Geometry check sheet. Reference: the model listing, model coordinates, mm. A direction names the side the tool comes from. Give positions to 0.01 mm unless a question says otherwise; leave off trailing zeros. Order: outer loops, then holes, each group sorted by start corner. A loop starts at its lowest first (then second) coordinate and runs counter-clockwise, first axis right, second up. Notation, with made-up numbers: M 54,33 L 84,33 A5 ccw 84,38 Z; hole C 19.5,1.25 d1. An arc over 180 degrees is marked long. Put each result on its own line as item: value. Start each with the question number.
Q1. Section check C-C on z = 10. State how many separate pieces and enclosed holes the cut face has, then the cut area to 3 significant figures.
Q2. Go/stop test with flat-tipped pins: pin 1 (10 mm diameter, centred on y = 134.5, z = 5, fed in from -X); pin 2 (8.5 mm diameter, centred on x = 9.5, y = 96, fed in from -Z). Record where each tip stops, or that it passes through.
Q3. Access from +Z, -Z, +X, -X, +Y, -Y to the whole of each face (thin tool, end or side, straight path). Record for faces 1 (the flat face through (89, 63, 10)), 2 (the flat face through (49, 0, 10)), 3 (the flat face through (49, 197.5, 9)).
Q4. Material ranges on L1, parallel to Y at x = 42.5, z = 14.5; L2, parallel to X at y = 33, z = 9.25; L3, parallel to X at y = 104.5, z = 6.5, recorded low to high.
Q5. Section check B-B on x = 72. Record the cut outline in (y, z).
Q6. Section check A-A on y = 178. Record the cut outline in (x, z), then the cut area to 3 significant figures.
Q7. Mould release check, pull along Z, two halves, no side actions. Record for faces 4 (the cylindrical face through (2.535, 37.754, 10.165)), 5 (the flat face through (16, 124, 20)), 6 (the flat face through (11, 63, 10)): +Z half, -Z half, draft (parallel to the pull), parting line (faces both ways), or undercut.
```python
from build123d import *

# Parameters (mm, degrees)
F0_W        = 100
F0_H        = 200
F0_W_2      = 12
F0_H_2      = 43
F0_W_3      = 56
F0_H_3      = 180
F1_DEPTH    = 20
F2_R        = 3.75
F3_DEPTH    = 100.001
F4_T        = 2.5
F4_T3_DEPTH = 25


# Not quite as in the source:
# - a shell that OpenCascade refuses in one call is made with other operations: the cavity is built on its own and cut out


with BuildPart() as f1:
    # F0 (on Top) → F1 (new body)
    with BuildSketch(Plane.XY):
        with Locations((50, 100)):
            Rectangle(F0_W, F0_H)
        with Locations((11, 41.5)):
            Rectangle(F0_W_2, F0_H_2, mode=Mode.SUBTRACT)
        Polygon((89, 20), (83, 20), (83, 63), (95, 63), (95, 20), align=None, mode=Mode.SUBTRACT)
        with Locations((11, 158.5)):
            Rectangle(F0_W_2, F0_H_2, mode=Mode.SUBTRACT)
        with Locations((50, 100)):
            Rectangle(F0_W_3, F0_H_3, mode=Mode.SUBTRACT)
        with Locations((89, 158.5)):
            Rectangle(F0_W_2, F0_H_2, mode=Mode.SUBTRACT)
    extrude(amount=F1_DEPTH)

    # F2 (on face) → F3 (cut, through all)
    with BuildSketch(Plane.YZ.offset(100)):
        with Locations((41.5, 10)):
            Circle(F2_R)
        with Locations((158.5, 10)):
            Circle(F2_R)
    extrude(amount=-F3_DEPTH, mode=Mode.SUBTRACT)

    # F4: shell of thickness 2.5, made by hand


with BuildPart() as f4_core1:
    # F4_t2: copy of F1
    add(f1.part)

    # the walls: a layer under each face that stays
    f4_faces = [f4_core1.faces().sort_by_distance(p)[0] for p in [
        (0, 100, 10),
        (50, 200, 10),
        (16.6666666667, 100, 20),
        (50, 0, 10),
        (2.5, 154.75, 10),
        (2.5, 37.75, 10),
        (100, 100, 10),
        (17, 55.8333333333, 16.6666666667),
        (11, 20, 10),
        (5, 27.1666666667, 16.6666666667),
        (11, 63, 10),
        (83, 27.1666666667, 16.6666666667),
        (89, 63, 10),
        (95, 55.8333333333, 16.6666666667),
        (89, 20, 10),
        (11, 180, 10),
        (17, 172.8333333333, 16.6666666667),
        (11, 137, 10),
        (5, 144.1666666667, 16.6666666667),
        (22, 100, 10),
        (50, 190, 10),
        (78, 100, 10),
        (50, 10, 10),
        (83, 144.1666666667, 16.6666666667),
        (89, 180, 10),
        (95, 172.8333333333, 16.6666666667),
        (89, 137, 10),
        (97.5, 37.75, 10),
        (97.5, 154.75, 10),
        (19.5, 37.75, 10),
        (80.5, 37.75, 10),
        (19.5, 154.75, 10),
        (80.5, 154.75, 10),
    ]]
    thicken(f4_faces, amount=-F4_T, mode=Mode.SUBTRACT)

    # F4_s4 → F4_t3 (cut)
    with BuildSketch(Plane.XY.offset(-2.5)):
        Polygon((16.975, 62.975), (19.5, 63), (19.5, 65.5), (17, 65.5), align=None)
        Polygon((16.975, 20.025), (19.5, 20), (19.5, 17.5), (17, 17.5), align=None)
        Polygon((5.025, 20.025), (5, 17.5), (2.5, 17.5), (2.5, 20), align=None)
        Polygon((5.025, 62.975), (2.5, 63), (2.5, 65.5), (5, 65.5), align=None)
        Polygon((83.025, 20.025), (80.5, 20), (80.5, 17.5), (83, 17.5), align=None)
        Polygon((83.025, 62.975), (80.5, 63), (80.5, 65.5), (83, 65.5), align=None)
        Polygon((94.975, 62.975), (95, 65.5), (97.5, 65.5), (97.5, 63), align=None)
        Polygon((94.975, 20.025), (97.5, 20), (97.5, 17.5), (95, 17.5), align=None)
        Polygon((5.025, 179.975), (5, 182.5), (2.5, 182.5), (2.5, 180), align=None)
        Polygon((16.975, 179.975), (17, 182.5), (19.5, 182.5), (19.5, 180), align=None)
        Polygon((16.975, 137.025), (19.5, 137), (19.5, 134.5), (17, 134.5), align=None)
        Polygon((5.025, 137.025), (5, 134.5), (2.5, 134.5), (2.5, 137), align=None)
        Polygon((22.025, 10.025), (19.5, 10), (19.5, 7.5), (22, 7.5), align=None)
        Polygon((22.025, 189.975), (19.5, 190), (19.5, 192.5), (22, 192.5), align=None)
        Polygon((77.975, 189.975), (78, 192.5), (80.5, 192.5), (80.5, 190), align=None)
        Polygon((77.975, 10.025), (80.5, 10), (80.5, 7.5), (78, 7.5), align=None)
        Polygon((83.025, 137.025), (80.5, 137), (80.5, 134.5), (83, 134.5), align=None)
        Polygon((83.025, 179.975), (80.5, 180), (80.5, 182.5), (83, 182.5), align=None)
        Polygon((94.975, 179.975), (95, 182.5), (97.5, 182.5), (97.5, 180), align=None)
        Polygon((94.975, 137.025), (97.5, 137), (97.5, 134.5), (95, 134.5), align=None)
    extrude(amount=F4_T3_DEPTH, mode=Mode.SUBTRACT)


with BuildPart() as f1_1:
    add(f1.part)

    # what is left inside the walls is the cavity
    f4_cavity = [f4_core1.part.solids().sort_by_distance(p)[0] for p in [
        (50, 197.475, 11.666667),
        (2.525, 100, 11.666667),
        (50, 2.525, 11.666667),
        (80.525, 100, 11.666667),
    ]]
    add(f4_cavity, mode=Mode.SUBTRACT)


solid = f1_1.part
```
Results found:
1. separate pieces: 4
1. enclosed holes: 4
1. area: 3,580 mm^2
2. pin 1: stops at x = 0
2. pin 2: stops at z = 17.5
3. face 1: +Z, -Z
3. face 2: +Z, -Z, +X, -X, -Y
3. face 3: -Z
4. L1: y = 0 to 2.5, 7.5 to 10, 190 to 192.5, 197.5 to 200
4. L2: x = 0 to 5, 17 to 22, 78 to 83, 95 to 100
4. L3: x = 0 to 2.5, 19.5 to 22, 78 to 80.5, 97.5 to 100
5. outline: M 0,0 L 2.5,0 L 2.5,17.5 L 7.5,17.5 L 7.5,0 L 10,0 L 10,20 L 0,20 Z; M 190,0 L 192.5,0 L 192.5,17.5 L 197.5,17.5 L 197.5,0 L 200,0 L 200,20 L 190,20 Z
6. outline: M 0,0 L 5,0 L 5,20 L 0,20 Z; M 17,0 L 22,0 L 22,20 L 17,20 Z; M 78,0 L 83,0 L 83,20 L 78,20 Z; M 95,0 L 100,0 L 100,20 L 95,20 Z
6. area: 400 mm^2
7. face 4: undercut
7. face 5: +Z half
7. face 6: draft
